Design review of the part built by this model. Coordinates are the model's own, in mm. Face numbers are marked on the shaded views. A direction names the side the tool comes from. Coordinates: 2 decimals unless noted, no trailing zeros. Answer as a JSON object with one key per item and string values.
from build123d import *

# Parameters (mm, degrees)
SKETCH1_R                = 20
SKETCH1_R_2              = 4
BOSS_EXTRUDE1_DEPTH      = 3
SKETCH3_R                = 15
CUT_EXTRUDE1_DEPTH       = 2.4
SKETCH4_R                = 2
CUT_EXTRUDE2_DEPTH       = 29.51245342
CIRPATTERN1_COUNT        = 5
BOSS_EXTRUDE3_DEPTH      = 1
BOSS_EXTRUDE3_DEPTH_BACK = 2
SKETCH14_R               = 5
SKETCH16_R               = 4
CUT_EXTRUDE3_DEPTH       = 29.655889447


with BuildPart() as part:
    # Sketch1 → Boss-Extrude1 (new, symmetric)
    with BuildSketch(Plane.XY):
        Circle(SKETCH1_R)
        Circle(SKETCH1_R_2, mode=Mode.SUBTRACT)
    extrude(amount=BOSS_EXTRUDE1_DEPTH, both=True)

    # Sketch3 → Cut-Extrude1 (cut)
    with BuildSketch(Plane.XY.offset(3)):
        Circle(SKETCH3_R)
    cut_extrude1 = extrude(amount=-CUT_EXTRUDE1_DEPTH, mode=Mode.SUBTRACT)

    # Mirror1: Cut-Extrude1 across plane
    add(cut_extrude1.mirror(Plane.XY), mode=Mode.SUBTRACT)

    # Sketch4 → Cut-Extrude2 (cut, through all)
    with BuildSketch(Plane.XY.offset(0.6)):
        with Locations((0, 9)):
            Circle(SKETCH4_R)
    cut_extrude2 = extrude(amount=-CUT_EXTRUDE2_DEPTH, mode=Mode.SUBTRACT)

    # CirPattern1: Cut-Extrude2 ×5 about axis
    cirpattern1_axis = Axis((0, 0, 0), (0, 0, 1))
    for i in range(1, CIRPATTERN1_COUNT):
        add(cut_extrude2.rotate(cirpattern1_axis, i * 360 / CIRPATTERN1_COUNT), mode=Mode.SUBTRACT)

    # Sketch5 → Cut-Revolve1 (revolve, cut)
    with BuildSketch(Plane(origin=(0, 0, 0), x_dir=(1, 0, 0), z_dir=(0, 1, 0))):
        Polygon((20, 2), (18.5, 1.133974596), (18.5, -1.133974596), (20, -2), align=None)
    revolve(axis=Axis((0, 0, 0), (0, 0, -1)), mode=Mode.SUBTRACT)

    # Sketch14 → Boss-Extrude3 (add, two sides: drawn at the far end of the back side and taken through both)
    with BuildSketch(Plane.XY.offset(0.6).offset(-BOSS_EXTRUDE3_DEPTH_BACK)):
        Circle(SKETCH14_R)
    extrude(amount=BOSS_EXTRUDE3_DEPTH + BOSS_EXTRUDE3_DEPTH_BACK)

    # Sketch16 → Cut-Extrude3 (cut, through all)
    with BuildSketch(Plane.XY.offset(1.6)):
        Circle(SKETCH16_R)
    extrude(amount=-CUT_EXTRUDE3_DEPTH, mode=Mode.SUBTRACT)


solid = part.part
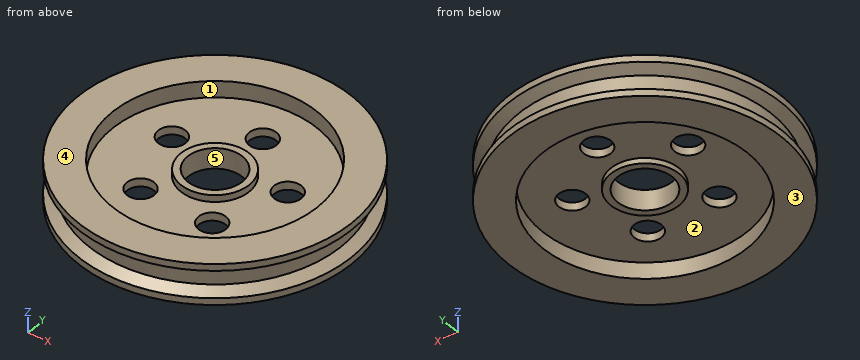
1) Tool access review of the marked faces 1, 2 and 3: name each direction out of +Z, -Z, +X, -X, +Y, -Y from which nothing blocks a thin tool from reaching the whole face with its end or side.
Taken from the geometry:
{"face 1": "+Z", "face 2": "-Z", "face 3": "-Z, +X, -X, +Y, -Y"}
2) To check wall thickness, follow L1, parallel to Y at x = 0, z = -0.2; L2, parallel to Y at x = 6, z = 2.35; L3, parallel to Y at x = -6.5, z = 1.8. State the ranges of each line that lie inside material, in increasing order.
Taken from the geometry:
{"L1": "y = -18.5 to -4, 4 to 7, 11 to 18.5", "L2": "y = -19.08 to -13.75, 13.75 to 19.08", "L3": "y = -18.55 to -13.52, 13.52 to 18.55"}
3) Mouldability with a two-part tool opening along X and no side actions: class the marked faces 4 and 5 as released by +X, released by -X, zero draft, split by the parting line, or undercut.
Taken from the geometry:
{"face 4": "zero draft", "face 5": "undercut"}
4) Insertion check: pin 1 Ø3 at (x, y) = (-5.29, -7.28) entering from -Z; pin 2 Ø8 at (x, y) = (-4, -5) entering from -Z; pin 3 Ø10.5 at (x, y) = (0, 0) entering from +Z; pin 4 Ø6.5 at (x, y) = (5.29, -7.28) entering from +Z. Each pin has a flat end and moves straight along its axis. Give the tip position at first contact, or say it passes through.
Taken from the geometry:
{"pin 1": "passes through", "pin 2": "stops at z = -1.4", "pin 3": "stops at z = 1.6", "pin 4": "stops at z = 0.6"}
5) Add section B-B (x = 0). Count the separate pieces of the cut face and the enclosed holes in it, and give its area (3 significant figures).
Taken from the geometry:
{"separate pieces": "3", "enclosed holes": "0", "area": "75.8 mm2"}
